```python
from build123d import *

# Parameters (mm, degrees)
REAR_LOCK_EAR_SKETCH_W             = 2
REAR_LOCK_EAR_SKETCH_H             = 22
REAR_LOCK_EAR_DEPTH                = 8
LOCK_FORK_WEB_SKETCH_W             = 11
LOCK_FORK_WEB_SKETCH_H             = 3
LOCK_FORK_WEB_DEPTH                = 30
FRONT_LOCK_EAR_SKETCH_W            = 2
FRONT_LOCK_EAR_SKETCH_H            = 22
FRONT_LOCK_EAR_DEPTH               = 8
FORK_MOUNTING_FOOT_SKETCH_W        = 11
FORK_MOUNTING_FOOT_SKETCH_H        = 22
FORK_MOUNTING_FOOT_DEPTH           = 2
COUPLING_BARREL_CLEARANCE_SKETCH_R = 6.3
COUPLING_BARREL_CLEARANCE_DEPTH    = 11.3
SERVICE_PIN_CLEARANCE_1_SKETCH_R   = 1.7
SERVICE_PIN_CLEARANCE_1_DEPTH      = 2.3
SERVICE_PIN_CLEARANCE_2_SKETCH_R   = 1.7
SERVICE_PIN_CLEARANCE_2_DEPTH      = 2.3
MOTOR_HEAD_ACCESS_1_1_SKETCH_R     = 3
MOTOR_HEAD_ACCESS_1_1_DEPTH        = 3.2
MOTOR_HEAD_ACCESS_1_5_SKETCH_R     = 3
MOTOR_HEAD_ACCESS_1_5_DEPTH        = 3.2
MOTOR_HEAD_ACCESS_2_1_SKETCH_R     = 3.05
MOTOR_HEAD_ACCESS_2_1_DEPTH        = 3.2
MOTOR_HEAD_ACCESS_2_5_SKETCH_R     = 3.05
MOTOR_HEAD_ACCESS_2_5_DEPTH        = 3.2


with BuildPart() as part:
    # Rear lock ear sketch → Rear lock ear (new body)
    with BuildSketch(Plane.XY.offset(-16)):
        with Locations((-11, -34)):
            Rectangle(REAR_LOCK_EAR_SKETCH_W, REAR_LOCK_EAR_SKETCH_H)
    extrude(amount=REAR_LOCK_EAR_DEPTH)

    # Lock fork web sketch → Lock fork web (add)
    with BuildSketch(Plane.XY.offset(-38)):
        with Locations((-6.5, -43.5)):
            Rectangle(LOCK_FORK_WEB_SKETCH_W, LOCK_FORK_WEB_SKETCH_H)
    extrude(amount=LOCK_FORK_WEB_DEPTH)

    # Front lock ear sketch → Front lock ear (add)
    with BuildSketch(Plane.XY.offset(-16)):
        with Locations((-2, -34)):
            Rectangle(FRONT_LOCK_EAR_SKETCH_W, FRONT_LOCK_EAR_SKETCH_H)
    extrude(amount=FRONT_LOCK_EAR_DEPTH)

    # Fork mounting foot sketch → Fork mounting foot (add)
    with BuildSketch(Plane.XY.offset(-38)):
        with Locations((-6.5, -34)):
            Rectangle(FORK_MOUNTING_FOOT_SKETCH_W, FORK_MOUNTING_FOOT_SKETCH_H)
    extrude(amount=FORK_MOUNTING_FOOT_DEPTH)

    # Coupling barrel clearance sketch → Coupling barrel clearance (cut)
    with BuildSketch(Plane(origin=(-12.1, 0, 0), x_dir=(0, 0, -1), z_dir=(1, 0, 0))):
        with Locations((19.5, -29)):
            Circle(COUPLING_BARREL_CLEARANCE_SKETCH_R)
    extrude(amount=COUPLING_BARREL_CLEARANCE_DEPTH, mode=Mode.SUBTRACT)

    # Service pin clearance 1 sketch → Service pin clearance 1 (cut)
    with BuildSketch(Plane(origin=(-12.1, 0, 0), x_dir=(0, 0, -1), z_dir=(1, 0, 0))):
        with Locations(Location((10.5, -29, 0), (0, 0, 180))):
            Circle(SERVICE_PIN_CLEARANCE_1_SKETCH_R)
    extrude(amount=SERVICE_PIN_CLEARANCE_1_DEPTH, mode=Mode.SUBTRACT)

    # Service pin clearance 2 sketch → Service pin clearance 2 (cut)
    with BuildSketch(Plane(origin=(-3.1, 0, 0), x_dir=(0, 0, -1), z_dir=(1, 0, 0))):
        with Locations(Location((10.5, -29, 0), (0, 0, 180))):
            Circle(SERVICE_PIN_CLEARANCE_2_SKETCH_R)
    extrude(amount=SERVICE_PIN_CLEARANCE_2_DEPTH, mode=Mode.SUBTRACT)

    # Motor head access 1-1 sketch → Motor head access 1-1 (cut)
    with BuildSketch(Plane(origin=(-12.1, 0, 0), x_dir=(0, 0, -1), z_dir=(1, 0, 0))):
        with Locations((34.765, -22.5)):
            Circle(MOTOR_HEAD_ACCESS_1_1_SKETCH_R)
    extrude(amount=MOTOR_HEAD_ACCESS_1_1_DEPTH, mode=Mode.SUBTRACT)

    # Motor head access 1-5 sketch → Motor head access 1-5 (cut)
    with BuildSketch(Plane(origin=(-12.1, 0, 0), x_dir=(0, 0, -1), z_dir=(1, 0, 0))):
        with Locations(Location((11.8675, -35.719877789, 0), (0, 0, 180))):
            Circle(MOTOR_HEAD_ACCESS_1_5_SKETCH_R)
    extrude(amount=MOTOR_HEAD_ACCESS_1_5_DEPTH, mode=Mode.SUBTRACT)

    # Motor head access 2-1 sketch → Motor head access 2-1 (cut)
    with BuildSketch(Plane(origin=(-12.1, 0, 0), x_dir=(0, 0, -1), z_dir=(1, 0, 0))):
        with Locations((35.25, -22)):
            Circle(MOTOR_HEAD_ACCESS_2_1_SKETCH_R)
    extrude(amount=MOTOR_HEAD_ACCESS_2_1_DEPTH, mode=Mode.SUBTRACT)

    # Motor head access 2-5 sketch → Motor head access 2-5 (cut)
    with BuildSketch(Plane(origin=(-12.1, 0, 0), x_dir=(0, 0, -1), z_dir=(1, 0, 0))):
        with Locations((11.625, -35.63990011)):
            Circle(MOTOR_HEAD_ACCESS_2_5_SKETCH_R)
    extrude(amount=MOTOR_HEAD_ACCESS_2_5_DEPTH, mode=Mode.SUBTRACT)


with BuildPart() as body_2:
    # Mirror1: mirrored copy
    add(part.part.mirror(Plane(origin=(0, 0, 0), x_dir=(0, 0, 1), z_dir=(0, -1, 0))))


solid = body_2.part
```
Check sheet for the modelled part. Datum: model origin and axes. Units: mm. A direction names the side the tool comes from. Round coordinates to 2 decimals unless told otherwise and drop trailing zeros. Order: outer loops, then holes, each group sorted by start corner. A loop starts at its lowest first (then second) coordinate and runs counter-clockwise, first axis right, second up. Notation, with made-up numbers: (-32, 20.25) -> (-17, 20.25) arc R13 cw to (-17, 26.25) -> close; hole circle Ø11 at (16, 51.25). An arc over 180 degrees is marked (long way). Use CSV: the item, a comma, the result in double quotes.
(1) Cross-section at D-D (z = -11). Record the boundary of the cut face in (x, y), and give its area (3 significant figures).
Worked out:
outline,"(-12, 23) -> (-10, 23) -> (-10, 27.38) -> (-12, 27.38) -> close; (-12, 30.62) -> (-10, 30.62) -> (-10, 32.65) -> (-12, 32.65) -> close; (-12, 38.63) -> (-10, 38.63) -> (-10, 42) -> (-3, 42) -> (-3, 30.62) -> (-1, 30.62) -> (-1, 45) -> (-12, 45) -> close; (-3, 23) -> (-1, 23) -> (-1, 27.38) -> (-3, 27.38) -> close"
area,"84.1 mm²"
(2) Cross-section at C-C (x = -10.5). Count the separate pieces of the cut face and the enclosed holes in it, and give its area (3 significant figures).
Worked out:
separate pieces,"1"
enclosed holes,"2"
area,"217 mm²"
(3) Material ranges on line 1 along Z through (x, y) = (-10.6, 29); line 2 along Z through (x, y) = (-1.5, 41); line 3 along Y through (x, z) = (-1.4, -10.5), recorded low to high. Write a range as from..to.
Worked out:
line 1,"-38..-36, -13.2..-12.2, -8.8..-8"
line 2,"-38..-36, -16..-8"
line 3,"23..27.3, 30.7..45"
(4) Draft check along X on faces 4 (the face through (-12, 42.2, -20.8)), 5 (the face through (-3, 35, -12)), 6 (the face through (-11, 28.9, -13.2)). Enter one of: pulls with the +X half, pulls with the -X half, needs draft (parallel to the pull), parting line crosses it, or undercut.
Worked out:
face 4,"pulls with the -X half"
face 5,"undercut"
face 6,"needs draft"
(5) Cross-section at B-B (x = -2). Record the boundary of the cut face in (y, z).
Worked out:
outline,"(23, -38) -> (45, -38) -> (45, -8) -> (23, -8) -> (23, -16) -> (23.76, -16) arc R6.3 cw to (34.24, -16) -> (42, -16) -> (42, -36) -> (23, -36) -> close; hole circle Ø3.4 at (29, -10.5)"
(6) Depth check by flat-ended pin: pin 1 (3 mm diameter, centred on x = -3.5, z = -34, fed in from -Y); pin 2 (3.5 mm diameter, centred on y = 35.64, z = -11.62, fed in from -X); pin 3 (2.5 mm diameter, centred on y = 29, z = -10.5, fed in from +X); pin 4 (0.6 mm diameter, centred on y = 23.5, z = -37.5, fed in from -X). Enter the tip coordinate at first touch or a pass-through.
Worked out:
pin 1,"y = 42"
pin 2,"x = -3"
pin 3,"through"
pin 4,"x = -8.9"
(7) Cross-section at A-A (y = 29). Record the boundary of the cut face in (x, z).
Worked out:
outline,"(-12, -38) -> (-1, -38) -> (-1, -36) -> (-12, -36) -> close; (-12, -13.2) -> (-10, -13.2) -> (-10, -12.2) -> (-12, -12.2) -> close; (-12, -8.8) -> (-10, -8.8) -> (-10, -8) -> (-12, -8) -> close; (-3, -13.2) -> (-1, -13.2) -> (-1, -12.2) -> (-3, -12.2) -> close; (-3, -8.8) -> (-1, -8.8) -> (-1, -8) -> (-3, -8) -> close"
(8) Tool access check on faces 1 (the face through (-10, 32.6, -12.9)), 2 (the face through (-8.9, 24, -37)), 3 (the face through (-10.47, 24.92, -36.54)). Record the directions out of +Z, -Z, +X, -X, +Y, -Y that give a thin tool (end or side, any length) a straight path to the whole face; none if there is none.
Worked out:
face 1,"+Z, -Y"
face 2,"+Z, -X, -Y"
face 3,"-X, -Y"
